Geometry: final body of the model. Coordinates: model frame, mm. Round coordinates to 2 decimals unless told otherwise and drop trailing zeros. Write each loop counter-clockwise with the first axis right and the second up, starting at its lowest first coordinate (ties: lowest second). Pieces come first, ordered by that corner, then holes. Notation, with made-up numbers: M -2.5,13.5 L 11.5,13.5 A24 cw 11.5,43.5 Z; hole C -8,-24.75 d7. An arc over 180 degrees is marked long. Answer as CSV lines item,"result". Start each with the question number.
Q1. Ray query, probe 1 along Z at (x, y) = (22, -2.25); probe 2 along Y at (x, z) = (17, 0.5); probe 3 along Z at (x, y) = (14.75, -2.5). Return the intervals inside material, ascending.
Q2. First-contact query: pin 1 (1 mm diameter, centred on x = 7.5, z = -2, fed in from +Y); pin 2 (3 mm diameter, centred on y = 2.5, z = 1.5, fed in from -X). Flat tips, straight axial feed; report the tip coordinate or a pass-through.
Q3. Section query A-A on x = 14. Output: boundary loops of the cut face in (y, z).
Autodesk Inventor part; units mm, degrees
ref_plane "Work Plane1" through (23.495, 0, 0) normal (1, 0, 0) x (0, 0, -1)
ref_plane "Work Plane2" through (-0.381, 0, 0) normal (-1, 0, 0) x (0, 0, 1)
ref_plane "YZ Plane" through (0, 0, 0) normal (1, 0, 0) x (0, 1, 0)
sketch "Sketch1" plane through (0, 0, 0) normal (1, 0, 0) x (0, 1, 0)
  circle A0 centre (0, 0) radius 3.048
  dimension "d0" = 6.096
extrude "Extrusion1" add sketch "Sketch1" along normal blind 23.114
ref_plane "Work Plane1" through (23.495, 0, 0) normal (1, 0, 0) x (0, 0, -1)
sketch "Sketch2" plane through (23.495, 0, 0) normal (1, 0, 0) x (0, 0, -1)
  circle A0 centre (0, 0) radius 2.54
  dimension "d4" = 5.08
loft "Loft1" add profiles "Sketch2" section 2 edges at (23.114, -3.048, 0)
ref_plane "Work Plane2" through (-0.381, 0, 0) normal (-1, 0, 0) x (0, 0, 1)
sketch "Sketch3" plane through (-0.381, 0, 0) normal (-1, 0, 0) x (0, 0, 1)
  circle A0 centre (0, 0) radius 2.54
  dimension "d10" = 5.08
loft "Loft2" add profiles "Sketch3" section 2 edges at (0, -3.048, 0)
properties part number "shaft 6x24-1"
Entries:
1,probe 1,"z = -2.06 to 2.06"
1,probe 2,"y = -3.01 to 3.01"
1,probe 3,"z = -1.74 to 1.74"
2,pin 1,"stops at y = 2.65"
2,pin 2,"stops at x = -0.38"
3,outline,"C 0,0 d6.1"
